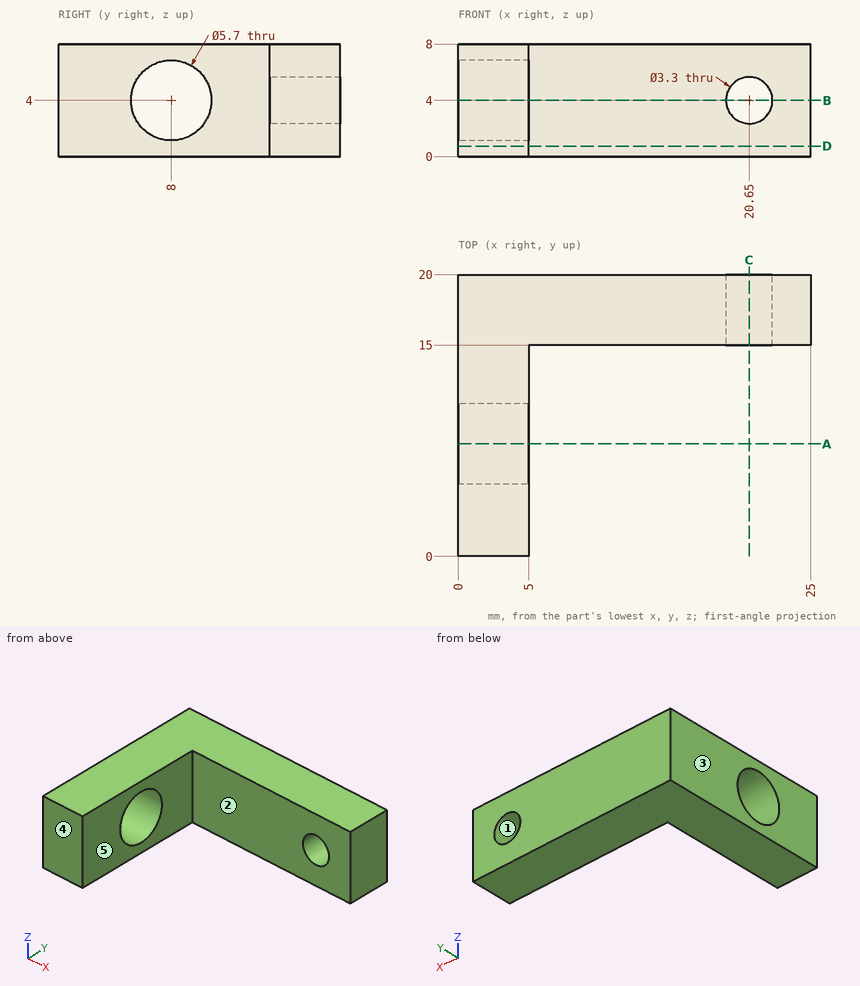
Answer from the drawing. Dimensions are ordinates in mm from the lowest x, y and z of the part. A direction names the side the tool comes from. Coordinates: 2 decimals unless noted, no trailing zeros. Write each loop counter-clockwise with the first axis right and the second up, starting at its lowest first coordinate (ties: lowest second). Pieces come first, ordered by that corner, then holes. Notation, with made-up numbers: (59.5, -13.5) - (107.5, -13.5) arc R18 cw to (107.5, 19.5) - close; hole circle Ø11 at (14.25, 57). An arc over 180 degrees is marked (long way). Return JSON: item names as keys, results as strings. Group by question number.
Q1. Which of the six approach directions +Z, -Z, +X, -X, +Y, -Y give full straight-line access (tool end or side, diameter ignored) to the marked faces 4 and 5?
Q2. The part is cut by section D-D on z = 0.75. Write down the section's boundary in (x, y).
Q3. Flat-ended cylindrical pins translate along their axes: pin 1 Ø4.5 at (x, z) = (20.65, 4) entering from +Y; pin 2 Ø2 at (y, z) = (4, 4) entering from +X; pin 3 Ø3.5 at (y, z) = (8, 4) entering from -X. Find the tip coordinate at first contact, or state that the pin passes through.
Q4. Find the intervals of material crossed by line 1 along Z through (x, y) = (2.05, 8); line 2 along Z through (x, y) = (20.65, 18.35); line 3 along Y through (x, z) = (5.25, 0.75), in increasing order. Write a range as [from, to].
Q5. The part is cut by section A-A on y = 8. Write down the section's boundary in (x, z).
Q6. The part is cut by section B-B on z = 4. Write down the section's boundary in (x, y), and give its area (3 significant figures).
Q7. The part is cut by section C-C on x = 20.65. Write down the section's boundary in (y, z).
Q8. For a pull along X with two mould halves and no side action, classify the marked faces 1, 2 and 3 as +X half, -X half, draft (parallel to the pull), parting line (faces both ways), or undercut.
Evaluation:
{
 "1": {"face 4": "+Z, -Z, +X, -X, -Y", "face 5": "+Z, -Z, +X, -Y"},
 "2": {"outline": "(0, 0) - (5, 0) - (5, 15) - (25, 15) - (25, 20) - (0, 20) - close"},
 "3": {"pin 1": "stops at y = 20", "pin 2": "stops at x = 5", "pin 3": "passes through"},
 "4": {"line 1": "z = [0, 1.15], [6.85, 8]", "line 2": "z = [0, 2.35], [5.65, 8]", "line 3": "y = [15, 20]"},
 "5": {"outline": "(0, 0) - (5, 0) - (5, 1.15) - (0, 1.15) - close; (0, 6.85) - (5, 6.85) - (5, 8) - (0, 8) - close"},
 "6": {"outline": "(0, 0) - (5, 0) - (5, 5.15) - (0, 5.15) - close; (0, 10.85) - (5, 10.85) - (5, 15) - (19, 15) - (19, 20) - (0, 20) - close; (22.3, 15) - (25, 15) - (25, 20) - (22.3, 20) - close", "area": "155 mm2"},
 "7": {"outline": "(15, 0) - (20, 0) - (20, 2.35) - (15, 2.35) - close; (15, 5.65) - (20, 5.65) - (20, 8) - (15, 8) - close"},
 "8": {"face 1": "undercut", "face 2": "draft", "face 3": "-X half"}
}
